```python
from build123d import *

# Parameters (mm, degrees)
F0_W     = 908.05
F0_H     = 127
F0_W_2   = 869.95
F0_H_2   = 88.9
F1_DEPTH = 730.25
F3_DEPTH = 25.4
F4_R     = 38.1
F5_DEPTH = 25.4


with BuildPart() as f1:
    # F0 (on Top) → F1 (new body)
    with BuildSketch(Plane.XY):
        Rectangle(F0_W, F0_H)
        Rectangle(F0_W_2, F0_H_2, mode=Mode.SUBTRACT)
    extrude(amount=F1_DEPTH)

    # F2 (on face) → F3 (cut)
    with BuildSketch(Plane.XZ.offset(63.5)):
        Polygon((-133.35, 101.6), (0, 101.6), (133.35, 101.6), (133.35, 419.1), (-133.35, 419.1), align=None)
    extrude(amount=-F3_DEPTH, mode=Mode.SUBTRACT)

    # F4 (on face) → F5 (cut)
    with BuildSketch(Plane.XZ.offset(63.5)):
        with Locations((0, 730.25)):
            Circle(F4_R)
    extrude(amount=-F5_DEPTH, mode=Mode.SUBTRACT)


solid = f1.part
```
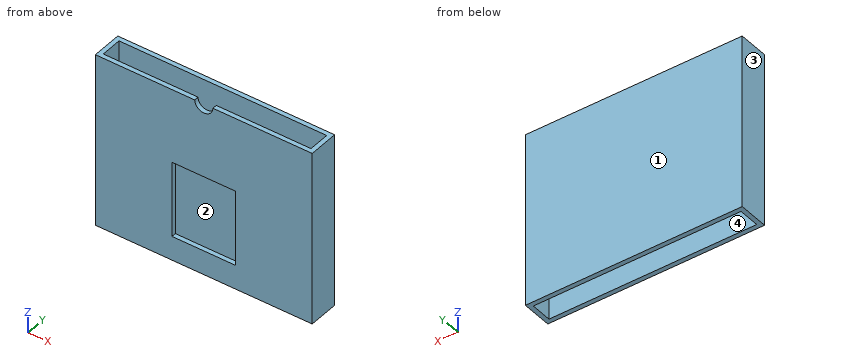
CAD build for the part. Positions are in the model's coordinates, mm. Face numbers are marked on the shaded views. Round coordinates to 2 decimals unless told otherwise and drop trailing zeros. Write each loop counter-clockwise with the first axis right and the second up, starting at its lowest first coordinate (ties: lowest second). Pieces come first, ordered by that corner, then holes. Notation, with made-up numbers: (-38.5, 64.5) -> (12.5, 64.5) arc R30 cw to (12.5, 98.5) -> close; hole circle Ø7 at (48, 27.25). An arc over 180 degrees is marked (long way). Answer in a Markdown table with one row per item. Add a question column.
Item 1: Mould opens along Y. For the marked faces 1, 2, 3 and 4 say: pulls with the +Y half, pulls with the -Y half, needs draft (parallel to the pull), parting line crosses it, or undercut.
Item 2: Saw through at C-C, the plane x = -241. Write the cut outline in (y, z).
Item 3: Saw through at D-D, the plane x = 0. Write the cut outline in (y, z), then the cut area to 3 significant figures.
Item 4: Saw through at B-B, the plane z = 621. Write the cut outline in (x, y) (3 decimals).
Item 5: Saw through at A-A, the plane y = -13. Write the cut outline in (x, z) (3 decimals), then the cut area to 3 significant figures.
Item 6: Drill centre lines: line 1 (X direction, y = -18.5, z = 410) (3 decimals); line 2 (Y direction, x = 168.5, z = 59); line 3 (X direction, y = -51.5, z = 408) (3 decimals). Where is each one in solid material? Low to high. Write a range as from..to.
Findings below:
| question | item | result |
|---|---|---|
| 1 | face 1 | pulls with the +Y half |
| 1 | face 2 | undercut |
| 1 | face 3 | needs draft |
| 1 | face 4 | undercut |
| 2 | outline | (-63.5, 0) -> (-44.45, 0) -> (-44.45, 730.25) -> (-63.5, 730.25) -> close; (44.45, 0) -> (63.5, 0) -> (63.5, 730.25) -> (44.45, 730.25) -> close |
| 3 | outline | (-63.5, 0) -> (-44.45, 0) -> (-44.45, 101.6) -> (-63.5, 101.6) -> close; (-63.5, 419.1) -> (-44.45, 419.1) -> (-44.45, 692.15) -> (-63.5, 692.15) -> close; (44.45, 0) -> (63.5, 0) -> (63.5, 730.25) -> (44.45, 730.25) -> close |
| 3 | area | 21,000 mm^2 |
| 4 | outline | (-454.025, -63.5) -> (454.025, -63.5) -> (454.025, 63.5) -> (-454.025, 63.5) -> close; hole (-434.975, -44.45) -> (434.975, -44.45) -> (434.975, 44.45) -> (-434.975, 44.45) -> close |
| 5 | outline | (-454.025, 0) -> (-434.975, 0) -> (-434.975, 730.25) -> (-454.025, 730.25) -> close; (434.975, 0) -> (454.025, 0) -> (454.025, 730.25) -> (434.975, 730.25) -> close |
| 5 | area | 27,800 mm^2 |
| 6 | line 1 | x = -454.025..-434.975, 434.975..454.025 |
| 6 | line 2 | y = -63.5..-44.45, 44.45..63.5 |
| 6 | line 3 | x = -454.025..-133.35, 133.35..454.025 |
